Source: three-view drawing plus pictorial views. Frame: mm from the lowest corner of the part. A direction names the side the tool comes from. Round coordinates to 2 decimals unless told otherwise and drop trailing zeros. Write each loop counter-clockwise with the first axis right and the second up, starting at its lowest first coordinate (ties: lowest second). Pieces come first, ordered by that corner, then holes. Notation, with made-up numbers: M 42,-33.5 L 99,-33.5 A16 ccw 99,-29.5 Z; hole C 44,8 d4. An arc over 180 degrees is marked long. Answer in a Markdown table with one row per item.
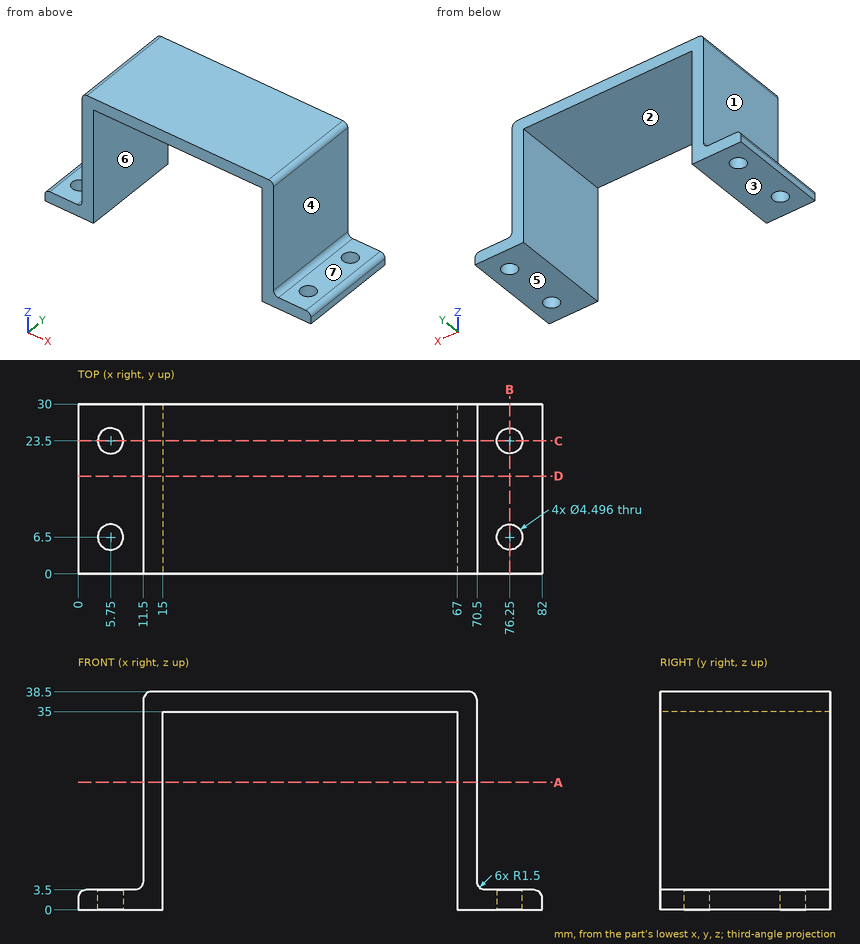
Q1. Section C-C (y = 23.5). Return loops of the section in (x, z).
Solutions:
| item | result |
|---|---|
| outline | M 0,0 L 3.5,0 L 3.5,3.5 L 1.5,3.5 A1.5 ccw 0,2 Z; M 8,0 L 15,0 L 15,35 L 67,35 L 67,0 L 74,0 L 74,3.5 L 72,3.5 A1.5 cw 70.5,5 L 70.5,37 A1.5 ccw 69,38.5 L 13,38.5 A1.5 ccw 11.5,37 L 11.5,5 A1.5 cw 10,3.5 L 8,3.5 Z; M 78.5,0 L 82,0 L 82,2 A1.5 ccw 80.5,3.5 L 78.5,3.5 Z |
Q2. Section D-D (y = 17.25). Return loops of the section in (x, z), and give its area (3 significant figures).
Solutions:
| item | result |
|---|---|
| outline | M 0,0 L 15,0 L 15,35 L 67,35 L 67,0 L 82,0 L 82,2 A1.5 ccw 80.5,3.5 L 72,3.5 A1.5 cw 70.5,5 L 70.5,37 A1.5 ccw 69,38.5 L 13,38.5 A1.5 ccw 11.5,37 L 11.5,5 A1.5 cw 10,3.5 L 1.5,3.5 A1.5 ccw 0,2 Z |
| area | 531 mm2 |
Q3. Section B-B (x = 76.25). Return loops of the section in (y, z).
Solutions:
| item | result |
|---|---|
| outline | M 0,0 L 4.25,0 L 4.25,3.5 L 0,3.5 Z; M 8.75,0 L 21.25,0 L 21.25,3.5 L 8.75,3.5 Z; M 25.75,0 L 30,0 L 30,3.5 L 25.75,3.5 Z |
Q4. Contact query for flat-ended pins moving along their axis: pin 1 Ø9 at (y, z) = (20, 22) entering from -X; pin 2 Ø9.5 at (x, y) = (7, 11) entering from +Z; pin 3 Ø9 at (y, z) = (21.5, 13.5) entering from +X; pin 4 Ø2.5 at (x, y) = (76.25, 6.5) entering from -Z. Output: stop coordinate, or through.
Solutions:
| item | result |
|---|---|
| pin 1 | stops at x = 11.5 |
| pin 2 | stops at z = 37.83 |
| pin 3 | stops at x = 70.5 |
| pin 4 | passes through |
Q5. Section A-A (z = 22.5). Return loops of the section in (x, y), and give its area (3 significant figures).
Solutions:
| item | result |
|---|---|
| outline | M 11.5,0 L 15,0 L 15,30 L 11.5,30 Z; M 67,0 L 70.5,0 L 70.5,30 L 67,30 Z |
| area | 210 mm2 |
Q6. Pull-direction query (X, two-part tool) for the marked faces 1, 2, 3 and 4; classes: pulls with the +X half, pulls with the -X half, needs draft (parallel to the pull), parting line crosses it, or undercut.
Solutions:
| item | result |
|---|---|
| face 1 | pulls with the -X half |
| face 2 | undercut |
| face 3 | needs draft |
| face 4 | pulls with the +X half |
Q7. Access query for the marked faces 5, 6 and 7. Directions: +Z, -Z, +X, -X, +Y, -Y. A direction counts if a zero-diameter tool reaches every point of the face in a straight line with its end or side. Return the directions, or none.
Solutions:
| item | result |
|---|---|
| face 5 | -Z, +X, -X, +Y, -Y |
| face 6 | -Z, +Y, -Y |
| face 7 | +Z, +X, +Y, -Y |
Q8. Material intervals for probe 1 along Y at (x, z) = (5.75, 1.15); probe 2 along X at (y, z) = (19, 14.5); probe 3 along Y at (x, z) = (5, 1), sorted ascending.
Solutions:
| item | result |
|---|---|
| probe 1 | y = 0 to 4.25, 8.75 to 21.25, 25.75 to 30 |
| probe 2 | x = 11.5 to 15, 67 to 70.5 |
| probe 3 | y = 0 to 4.38, 8.62 to 21.38, 25.62 to 30 |
